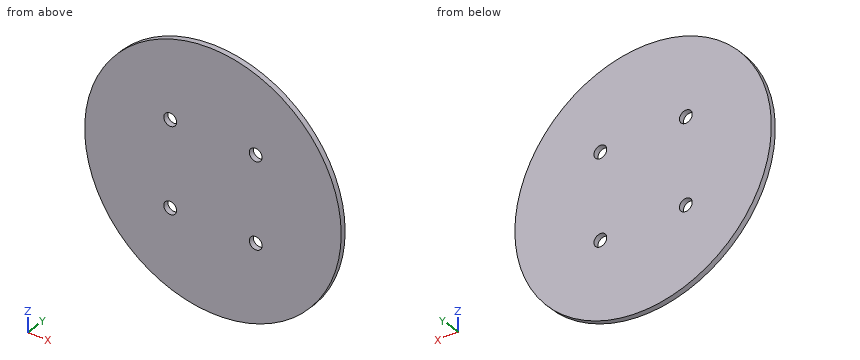
from build123d import *

# Parameters (mm, degrees)
SKETCH1_R           = 76.2
SKETCH1_R_2         = 3.81
BOSS_EXTRUDE1_DEPTH = 3.175


with BuildPart() as part:
    # Sketch1 → Boss-Extrude1 (new body)
    with BuildSketch(Plane(origin=(0, 0, 0), x_dir=(1, 0, 0), z_dir=(0, 1, 0))):
        Circle(SKETCH1_R)
        with Locations((-25.4, 25.4)):
            Circle(SKETCH1_R_2, mode=Mode.SUBTRACT)
        with Locations((-25.4, -25.4)):
            Circle(SKETCH1_R_2, mode=Mode.SUBTRACT)
        with Locations((25.4, -25.4)):
            Circle(SKETCH1_R_2, mode=Mode.SUBTRACT)
        with Locations((25.4, 25.4)):
            Circle(SKETCH1_R_2, mode=Mode.SUBTRACT)
    extrude(amount=BOSS_EXTRUDE1_DEPTH)


solid = part.part
Geometry: final body of the model. Coordinates: model frame, mm. Coordinates: 2 decimals unless noted, no trailing zeros. Order: outer loops, then holes, each group sorted by start corner. A loop starts at its lowest first (then second) coordinate and runs counter-clockwise, first axis right, second up.
1) Ray query, probe 1 along Z at (x, y) = (25.4, 1.4); probe 2 along X at (y, z) = (1.75, -26.5); probe 3 along Z at (x, y) = (28.5, 0.7). Return the intervals inside material, ascending.
Result sheet:
probe 1: z = -71.84 to -29.21, -21.59 to 21.59, 29.21 to 71.84
probe 2: x = -71.44 to -29.05, -21.75 to 21.75, 29.05 to 71.44
probe 3: z = -70.67 to -27.61, -23.19 to 23.19, 27.61 to 70.67
2) First-contact query: P1, Ø1.5, axis at x = -31, y = 0.5, coming from the -Z side; P2, Ø7, axis at x = 25.4, z = -25.4, coming from the +Y side; P3, Ø1.5, axis at x = 59, y = 1.5, coming from the -Z side. Flat tips, straight axial feed; report the tip coordinate or a pass-through.
Result sheet:
P1: stops at z = -69.94
P2: passes through
P3: stops at z = -49.13
3) Section B-B (y = 1). Return loops of the section in (x, z), then the cut area to 3 significant figures.
Result sheet:
outline: circle Ø152.4 at (0, 0); hole circle Ø7.62 at (-25.4, -25.4); hole circle Ø7.62 at (-25.4, 25.4); hole circle Ø7.62 at (25.4, -25.4); hole circle Ø7.62 at (25.4, 25.4)
area: 18,100 mm2
4) Section D-D (z = -54). Return loops of the section in (x, y) (3 decimals).
Result sheet:
outline: (-53.763, 0) - (53.763, 0) - (53.763, 3.175) - (-53.763, 3.175) - close
5) Section C-C (z = -25.4). Return loops of the section in (x, y) (3 decimals), then the cut area to 3 significant figures.
Result sheet:
outline: (-71.842, 0) - (-29.21, 0) - (-29.21, 3.175) - (-71.842, 3.175) - close; (-21.59, 0) - (21.59, 0) - (21.59, 3.175) - (-21.59, 3.175) - close; (29.21, 0) - (71.842, 0) - (71.842, 3.175) - (29.21, 3.175) - close
area: 408 mm2
6) Section A-A (x = 25.4). Return loops of the section in (y, z) (3 decimals), then the cut area to 3 significant figures.
Result sheet:
outline: (0, -71.842) - (3.175, -71.842) - (3.175, -29.21) - (0, -29.21) - close; (0, -21.59) - (3.175, -21.59) - (3.175, 21.59) - (0, 21.59) - close; (0, 29.21) - (3.175, 29.21) - (3.175, 71.842) - (0, 71.842) - close
area: 408 mm2
